Work out the finished part from the listing and answer in its coordinate system (mm). A direction names the side the tool comes from. Give positions to 0.01 mm unless a question says otherwise; leave off trailing zeros. Order: outer loops, then holes, each group sorted by start corner. A loop starts at its lowest first (then second) coordinate and runs counter-clockwise, first axis right, second up. Notation, with made-up numbers: M 39,-26 L 81,-26 A7 ccw 81,-18 Z; hole C -39,51 d10. An arc over 180 degrees is marked long. One line per item, written item: value.
from build123d import *

# Parameters (mm, degrees)
F0_R     = 1
F1_DEPTH = 3


with BuildPart() as f1:
    # F0 (on Front) → F1 (new body)
    with BuildSketch(Plane.XZ):
        Polygon((-20, 0), (0, 0), (0, 7), (-3, 7), (-3, 17), (0, 17), (0, 24), (-3, 24), (-3, 34), (0, 34), (0, 41), (-20, 41), (-20, 38), (-30, 38), (-30, 41), (-50, 41), (-50, 38), (-55, 38), (-60, 38), (-60, 41), (-80, 41), (-80, 38), (-90, 38), (-90, 41), (-110, 41), (-110, 34), (-107, 34), (-107, 24), (-110, 24), (-110, 17), (-107, 17), (-107, 7), (-110, 7), (-110, 0), (-90, 0), (-90, 3), (-80, 3), (-80, 0), (-60, 0), (-60, 3), (-55, 3), (-50, 3), (-50, 0), (-30, 0), (-30, 3), (-20, 3), align=None)
        with Locations((-70, 1.5)):
            Circle(F0_R, mode=Mode.SUBTRACT)
        with Locations((-40, 1.5)):
            Circle(F0_R, mode=Mode.SUBTRACT)
        with Locations((-108.5, 20.5)):
            Circle(F0_R, mode=Mode.SUBTRACT)
        with Locations((-70, 39.5)):
            Circle(F0_R, mode=Mode.SUBTRACT)
        with Locations((-1.5, 20.5)):
            Circle(F0_R, mode=Mode.SUBTRACT)
        with Locations((-40, 39.5)):
            Circle(F0_R, mode=Mode.SUBTRACT)
    extrude(amount=F1_DEPTH)


solid = f1.part
(1) Find the intervals of material crossed by probe 1 along Z at (x, y) = (-1.5, -2.25); probe 2 along Z at (x, y) = (-70, -1.5); probe 3 along X at (y, z) = (-1.65, 16.5), in increasing order. Write a range as from..to.
Findings:
probe 1: z = 0..7, 17..19.5, 21.5..24, 34..41
probe 2: z = 0..0.5, 2.5..38.5, 40.5..41
probe 3: x = -107..-3
(2) Section A-A, the plane z = 20.5 is taken. Give the vertices of the cut face in (x, y).
Findings:
outline: M -110,-3 L -109.5,-3 L -109.5,0 L -110,0 Z; M -107.5,-3 L -2.5,-3 L -2.5,0 L -107.5,0 Z; M -0.5,-3 L 0,-3 L 0,0 L -0.5,0 Z
(3) Section D-D, the plane x = -108.5 is taken. Give the vertices of the cut face in (y, z), then the cut area to 3 significant figures.
Findings:
outline: M -3,0 L 0,0 L 0,7 L -3,7 Z; M -3,17 L 0,17 L 0,19.5 L -3,19.5 Z; M -3,21.5 L 0,21.5 L 0,24 L -3,24 Z; M -3,34 L 0,34 L 0,41 L -3,41 Z
area: 57.0 mm^2
(4) Which of the six approach directions +Z, -Z, +X, -X, +Y, -Y give full straight-line access (tool end or side, diameter ignored) to faces 1 (the flat face through (-50, -1, 2)), 2 (the flat face through (-1, -1, 24)), 3 (the flat face through (-108, -1, 24))?
Findings:
face 1: -Z, +Y, -Y
face 2: +X, +Y, -Y
face 3: -X, +Y, -Y
(5) Section C-C, the plane z = 39.5 is taken. Give the vertices of the cut face in (x, y), then the cut area to 3 significant figures.
Findings:
outline: M -110,-3 L -90,-3 L -90,0 L -110,0 Z; M -80,-3 L -71,-3 L -71,0 L -80,0 Z; M -69,-3 L -60,-3 L -60,0 L -69,0 Z; M -50,-3 L -41,-3 L -41,0 L -50,0 Z; M -39,-3 L -30,-3 L -30,0 L -39,0 Z; M -20,-3 L 0,-3 L 0,0 L -20,0 Z
area: 228 mm^2
(6) Section B-B, the plane x = -70 is taken. Give the vertices of the cut face in (y, z), then the cut area to 3 significant figures.
Findings:
outline: M -3,0 L 0,0 L 0,0.5 L -3,0.5 Z; M -3,2.5 L 0,2.5 L 0,38.5 L -3,38.5 Z; M -3,40.5 L 0,40.5 L 0,41 L -3,41 Z
area: 111 mm^2
(7) Determine the mould class of faces 4 (the flat face through (-40, -1, 0)), 5 (the flat face through (-108, -1, 7)), 6 (the flat face through (-50, -1, 40)), 7 (the flat face through (-40, -1, 41)) for opening direction Z: pulls with the +Z half, pulls with the -Z half, needs draft (parallel to the pull), parting line crosses it, or undercut.
Findings:
face 4: pulls with the -Z half
face 5: undercut
face 6: needs draft
face 7: pulls with the +Z half
(8) Given P1, Ø1.8, axis at x = -108.5, z = 20.5, coming from the +Y side; P2, Ø1, axis at y = -1.5, z = 10, coming from the +X side; P3, Ø0.9, axis at x = -26.5, y = -1.5, coming from the -Z side, each flat-ended and moving along its own axis, determine where each tip first touches the part or whether it passes through.
Findings:
P1: passes through
P2: stops at x = -3
P3: stops at z = 3
